```python
from build123d import *

# Parameters (mm, degrees)
SKETCH_1_R          = 11
SKETCH_1_R_2        = 4
EXTRUDE_1_DEPTH     = 3.5
CHAMFER_1_SIZE      = 0.5
SKETCH_2_R          = 9.6
SKETCH_2_R_2        = 6.05
CUT_EXTRUDE_1_DEPTH = 0.5


with BuildPart() as part:
    # 스케치1 → 보스-돌출1 (new, symmetric)
    with BuildSketch(Plane.XY):
        Circle(SKETCH_1_R)
        Circle(SKETCH_1_R_2, mode=Mode.SUBTRACT)
    extrude(amount=EXTRUDE_1_DEPTH, both=True)

    # 모따기1
    chamfer_1_edges = [part.edges().sort_by_distance(p)[0] for p in [
        (-11, 0, -3.5),
        (-11, 0, 3.5),
    ]]
    chamfer(chamfer_1_edges, length=CHAMFER_1_SIZE)

    # 스케치2 → 컷-돌출1 (cut)
    with BuildSketch(Plane.XY.offset(3.5)):
        Circle(SKETCH_2_R)
        Circle(SKETCH_2_R_2, mode=Mode.SUBTRACT)
    cut_extrude_1 = extrude(amount=-CUT_EXTRUDE_1_DEPTH, mode=Mode.SUBTRACT)

    # 대칭 복사1: 컷-돌출1 across plane
    add(cut_extrude_1.mirror(Plane.XY), mode=Mode.SUBTRACT)


solid = part.part
```
Verification items for the finished model (mm, model axes). A direction names the side the tool comes from. Give positions to 0.01 mm unless a question says otherwise; leave off trailing zeros. Order: outer loops, then holes, each group sorted by start corner. A loop starts at its lowest first (then second) coordinate and runs counter-clockwise, first axis right, second up. Notation, with made-up numbers: M 24.25,-24 L 36.25,-24 A23 cw 36.25,15 Z; hole C 43.25,-30.5 d10. An arc over 180 degrees is marked long. Return JSON: item names as keys, results as strings. Group by question number.
1) Section check C-C on z = -0.5. Record the cut outline in (x, y), and give its area (3 significant figures).
2) Mould release check, pull along X, two halves, no side actions. Record for faces 1 (the face through (5, -9, -3.5)), 2 (the face through (-2.38, -10.74, 0.04)), 3 (the face through (-0.1, -6.3, -3)): pulls with the +X half, pulls with the -X half, needs draft (parallel to the pull), parting line crosses it, or undercut.
3) Section check A-A on x = 0. Record the cut outline in (y, z).
4) Scan lines: line 1 (Y direction, x = 0, z = -1.5); line 2 (Y direction, x = 0, z = -3.3); line 3 (Z direction, x = 2.75, y = -8). Record each from-to range of solid material in increasing order.
5) Access from +Z, -Z, +X, -X, +Y, -Y to the whole of each face (thin tool, end or side, straight path). Record for faces 4 (the face through (-0.1, -6.3, 3)), 5 (the face through (-1.43, -3.95, -3.5)), 6 (the face through (5.161, 8.095, -3.254)).
6) Go/stop test with flat-tipped pins: pin 1 Ø4 at (y, z) = (-6, -0.5) entering from +X; pin 2 Ø2 at (x, z) = (-6.5, -2.5) entering from +Y; pin 3 Ø1 at (x, y) = (1.5, 7.5) entering from -Z. Record where each tip stops, or that it passes through.
Answer block:
{
 "1": {"outline": "C 0,0 d22; hole C 0,0 d8", "area": "330 mm^2"},
 "2": {"face 1": "needs draft", "face 2": "parting line crosses it", "face 3": "undercut"},
 "3": {"outline": "M -11,-3 L -10.5,-3.5 L -9.6,-3.5 L -9.6,-3 L -6.05,-3 L -6.05,-3.5 L -4,-3.5 L -4,3.5 L -6.05,3.5 L -6.05,3 L -9.6,3 L -9.6,3.5 L -10.5,3.5 L -11,3 Z; M 4,-3.5 L 6.05,-3.5 L 6.05,-3 L 9.6,-3 L 9.6,-3.5 L 10.5,-3.5 L 11,-3 L 11,3 L 10.5,3.5 L 9.6,3.5 L 9.6,3 L 6.05,3 L 6.05,3.5 L 4,3.5 Z"},
 "4": {"line 1": "y = -11 to -4, 4 to 11", "line 2": "y = -10.7 to -9.6, -6.05 to -4, 4 to 6.05, 9.6 to 10.7", "line 3": "z = -3 to 3"},
 "5": {"face 4": "+Z", "face 5": "-Z, +X, -X, +Y, -Y", "face 6": "-Z"},
 "6": {"pin 1": "stops at x = 10.25", "pin 2": "stops at y = 9.53", "pin 3": "stops at z = -3"}
}
